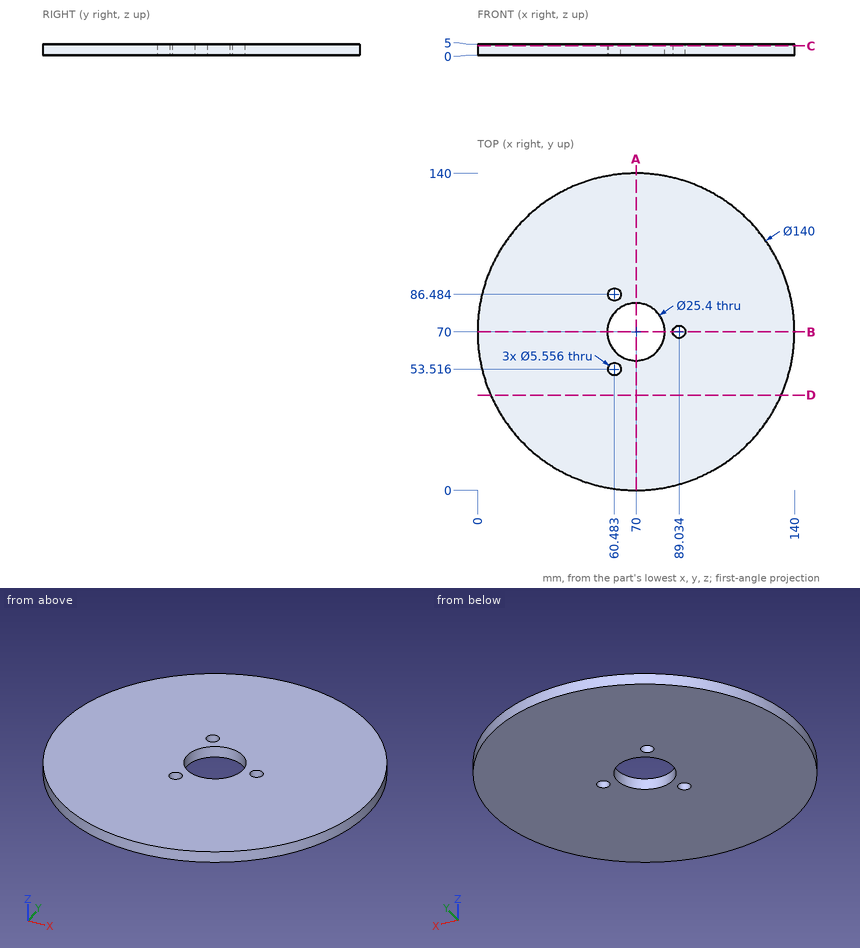
Verification items for this drawing (mm, ordinates from the low corner). Give positions to 0.01 mm unless a question says otherwise; leave off trailing zeros. Write each loop counter-clockwise with the first axis right and the second up, starting at its lowest first coordinate (ties: lowest second). Pieces come first, ordered by that corner, then holes.
1) Section check B-B, the plane y = 70. Record the boundary of the cut face in (x, z), and give its area (3 significant figures).
2) Section check A-A, the plane x = 70. Record the boundary of the cut face in (y, z), and give its area (3 significant figures).
3) Material ranges on L1, parallel to Y at x = 70, z = 1.8; L2, parallel to Y at x = 76.5, z = 1.8; L3, parallel to X at y = 58.5, z = 3.15, recorded low to high.
4) Section check D-D, the plane y = 42. Record the boundary of the cut face in (x, z).
5) Gauge pin test, flat ends, axial feed: pin 1 (1.5 mm diameter, centred on x = 61.5, z = 3.5, fed in from +Y); pin 2 (4.5 mm diameter, centred on x = 60.48, y = 53.52, fed in from -Z); pin 3 (1.5 mm diameter, centred on x = 117.5, z = 4, fed in from -Y); pin 4 (2 mm diameter, centred on x = 31.5, z = 1.5, fed in from -Y). Record the tip position at first contact, or that the pin passes through.
6) Section check C-C, the plane z = 4.2. Record the boundary of the cut face in (x, y), and give its area (3 significant figures).
Computed:
1. outline: (0, 0) - (57.3, 0) - (57.3, 5) - (0, 5) - close; (82.7, 0) - (86.26, 0) - (86.26, 5) - (82.7, 5) - close; (91.81, 0) - (140, 0) - (140, 5) - (91.81, 5) - close
1. area: 545 mm2
2. outline: (0, 0) - (57.3, 0) - (57.3, 5) - (0, 5) - close; (82.7, 0) - (140, 0) - (140, 5) - (82.7, 5) - close
2. area: 573 mm2
3. L1: y = 0 to 57.3, 82.7 to 140
3. L2: y = 0.3 to 59.09, 80.91 to 139.7
3. L3: x = 0.95 to 64.61, 75.39 to 139.05
4. outline: (5.84, 0) - (134.16, 0) - (134.16, 5) - (5.84, 5) - close
5. pin 1: stops at y = 139.57
5. pin 2: passes through
5. pin 3: stops at y = 17.9
5. pin 4: stops at y = 10.89
6. outline: circle Ø140 at (70, 70); hole circle Ø25.4 at (70, 70); hole circle Ø5.56 at (60.48, 53.52); hole circle Ø5.56 at (60.48, 86.48); hole circle Ø5.56 at (89.03, 70)
6. area: 14,800 mm2
